Check sheet for the modelled part. Datum: model origin and axes. Units: mm. A direction names the side the tool comes from. Coordinates: 2 decimals unless noted, no trailing zeros. Order: outer loops, then holes, each group sorted by start corner. A loop starts at its lowest first (then second) coordinate and runs counter-clockwise, first axis right, second up. Notation, with made-up numbers: M -35.5,72.25 L -19.5,72.25 A21 cw -19.5,76.25 Z; hole C -17.75,64.25 d11. An arc over 180 degrees is marked long. Answer in a Markdown table with one row per item. Add a question column.
from build123d import *

# Parameters (mm, degrees)
EXTRUDE_1_DEPTH              = 8
FILLET_1_R                   = 30
SKETCH_2_R                   = 14
CUT_EXTRUDE_1_DEPTH          = 4
HOLE_WIZARD_M4_1_D           = 4.5
HOLE_WIZARD_M3_1_D           = 3.4
HOLE_WIZARD_M3_1_DEPTH       = 8
HOLE_WIZARD_M3_1_CSINK_D     = 6.72
HOLE_WIZARD_M3_1_CSINK_ANGLE = 90
HOLE_WIZARD_M3_1_2_D         = 2.5
HOLE_WIZARD_M3_1_2_DEPTH     = 8.5
HOLE_WIZARD_M3_1_2_TIP       = 0.751075774


with BuildPart() as part:
    # 스케치1 → 보스-돌출1 (new body)
    with BuildSketch(Plane.XY):
        with BuildLine():
            Line((0, 35), (0, 0))
            Line((0, 0), (50, 0))
            Line((50, 0), (50, 35))
            Line((50, 35), (43.670126691, 68.525105576))
            ThreePointArc((43.670126691, 68.525105576), (25, 84), (6.329873309, 68.525105576))
            Line((6.329873309, 68.525105576), (0, 35))
        make_face()
    extrude(amount=EXTRUDE_1_DEPTH)

    # 필렛1
    fillet_1_edges = [part.edges().sort_by_distance(p)[0] for p in [
        (50, 35, 4),
        (0, 35, 4),
    ]]
    fillet(fillet_1_edges, radius=FILLET_1_R)

    # 스케치2 → 컷-돌출1 (cut)
    with BuildSketch(Plane(origin=(0, 0, 0), x_dir=(-1, 0, 0), z_dir=(0, 0, -1))):
        with Locations((-25, 65)):
            Circle(SKETCH_2_R)
    extrude(amount=-CUT_EXTRUDE_1_DEPTH, mode=Mode.SUBTRACT)

    # M4 여유 구멍1 (through all)
    with Locations(Plane.XY.offset(8)):
        with Locations((25, 65)):
            Hole(HOLE_WIZARD_M4_1_D / 2)

    # Hole Wizard M3 _ _ _ _ _ _ _1
    with Locations(Plane.XY.offset(8)):
        with Locations((4, 16), (4, 4), (46, 4), (46, 16)):
            CounterSinkHole(HOLE_WIZARD_M3_1_D / 2, HOLE_WIZARD_M3_1_CSINK_D / 2, depth=HOLE_WIZARD_M3_1_DEPTH, counter_sink_angle=HOLE_WIZARD_M3_1_CSINK_ANGLE)

    # Hole Wizard M3 _ _1 2
    with Locations(Plane(origin=(0, 0, 0), x_dir=(-1, 0, 0), z_dir=(0, -1, 0))):
        with Locations((-38, -4), (-12, -4)):
            Hole(HOLE_WIZARD_M3_1_2_D / 2, depth=HOLE_WIZARD_M3_1_2_DEPTH)
            with Locations((0, 0, -(HOLE_WIZARD_M3_1_2_DEPTH + HOLE_WIZARD_M3_1_2_TIP / 2))):  # 118° drill point
                Cone(0, HOLE_WIZARD_M3_1_2_D / 2, HOLE_WIZARD_M3_1_2_TIP, mode=Mode.SUBTRACT)


solid = part.part
1. Scan lines: line 1 (X direction, y = 16, z = 4.5); line 2 (Z direction, x = 12, y = 3.25); line 3 (X direction, y = 2.5, z = 4). Record each from-to range of solid material in increasing order.
2. Section check C-C on x = 4. Enter the section's corners in (y, z).
3. Section check B-B on y = 4. Enter the section's corners in (x, z).
4. Release check for a two-part mould opening along X. For faces 4 (the conical face through (12.028, 9.121, 3.785)), 5 (the flat face through (46.615, 52.926, 3.944)), 6 (the flat face through (3.466, 53.357, 3.944)) record: released by +X, released by -X, zero draft, split by the parting line, or undercut.
5. Section check A-A on x = 25. Enter the section's corners in (y, z).
6. Section check D-D on y = 66. Enter the section's corners in (x, z), then the cut area to 3 significant figures.
7. Go/stop test with flat-tipped pins: pin 1 Ø3 at (y, z) = (54.5, 7) entering from -X; pin 2 Ø4 at (x, y) = (4, 16) entering from +Z; pin 3 Ø22.5 at (x, y) = (25, 65) entering from -Z; pin 4 Ø3 at (x, y) = (46, 16) entering from +Z. Record where each tip stops, or that it passes through.
8. Set-up check for faces 1 (the flat face through (0, 16, 4)), 2 (the cylindrical face through (11.01, 4.31, 4.76)), 3 (the cylindrical face through (26.82, 78.88, 1.97)): record each of +Z, -Z, +X, -X, +Y, -Y from which the full face is reachable in a straight line by a thin tool's end or side.
Result sheet:
| question | item | result |
|---|---|---|
| 1 | line 1 | 0 to 2.3, 5.7 to 44.3, 47.7 to 50 |
| 1 | line 2 | 0 to 2.75, 5.25 to 8 |
| 1 | line 3 | 0 to 3.2, 4.8 to 10.75, 13.25 to 36.75, 39.25 to 45.2, 46.8 to 50 |
| 2 | outline | M 0,0 L 2.3,0 L 2.3,6.34 L 0.64,8 L 0,8 Z; M 5.7,0 L 14.3,0 L 14.3,6.34 L 12.64,8 L 7.36,8 L 5.7,6.34 Z; M 17.7,0 L 56.19,0 L 56.19,8 L 19.36,8 L 17.7,6.34 Z |
| 3 | outline | M 0,0 L 2.3,0 L 2.3,6.34 L 0.64,8 L 0,8 Z; M 5.7,0 L 44.3,0 L 44.3,6.34 L 42.64,8 L 7.36,8 L 5.7,6.34 Z; M 47.7,0 L 50,0 L 50,8 L 49.36,8 L 47.7,6.34 Z; hole C 12,4 d2.5; hole C 38,4 d2.5 |
| 4 | face 4 | undercut |
| 4 | face 5 | released by +X |
| 4 | face 6 | released by -X |
| 5 | outline | M 0,0 L 51,0 L 51,4 L 62.75,4 L 62.75,8 L 0,8 Z; M 67.25,4 L 79,4 L 79,0 L 84,0 L 84,8 L 67.25,8 Z |
| 6 | outline | M 5.85,0 L 11.04,0 L 11.04,4 L 22.98,4 L 22.98,8 L 5.85,8 Z; M 27.02,4 L 38.96,4 L 38.96,0 L 44.15,0 L 44.15,8 L 27.02,8 Z |
| 6 | area | 179 mm^2 |
| 7 | pin 1 | x = 3.4 |
| 7 | pin 2 | z = 6.64 |
| 7 | pin 3 | z = 4 |
| 7 | pin 4 | through |
| 8 | face 1 | +Z, -Z, -X, +Y, -Y |
| 8 | face 2 | -Y |
| 8 | face 3 | -Z |
